```python
from build123d import *

# Parameters (mm, degrees)
SKETCH1_W           = 210
SKETCH1_H           = 210
SKETCH1_R           = 1.5
SKETCH1_R_2         = 10
SKETCH1_R_3         = 1.25
SKETCH1_W_2         = 30
SKETCH1_H_2         = 6.134133664
SKETCH1_H_3         = 6
SKETCH1_W_3         = 6.572229622
SKETCH1_H_4         = 24
SKETCH1_W_4         = 6
BOSS_EXTRUDE1_DEPTH = 6


with BuildPart() as part:
    # Sketch1 → Boss-Extrude1 (new body)
    with BuildSketch(Plane(origin=(0, 0, 0), x_dir=(1, 0, 0), z_dir=(0, 1, 0))):
        with Locations((-0.850910849, -4.383508225)):
            Rectangle(SKETCH1_W, SKETCH1_H)
        with Locations((-98.850910849, -90.383508225)):
            Circle(SKETCH1_R, mode=Mode.SUBTRACT)
        with Locations((-87.850910849, -90.383508225)):
            Circle(SKETCH1_R, mode=Mode.SUBTRACT)
        with Locations((-0.850910849, -60.383508225)):
            Circle(SKETCH1_R_2, mode=Mode.SUBTRACT)
        with Locations((-87.850910849, -30.383508225)):
            Circle(SKETCH1_R, mode=Mode.SUBTRACT)
        with Locations((-98.850910849, -30.383508225)):
            Circle(SKETCH1_R, mode=Mode.SUBTRACT)
        with Locations((97.149089151, -90.383508225)):
            Circle(SKETCH1_R, mode=Mode.SUBTRACT)
        with Locations((86.149089151, -90.383508225)):
            Circle(SKETCH1_R, mode=Mode.SUBTRACT)
        with Locations((86.149089151, -30.383508225)):
            Circle(SKETCH1_R, mode=Mode.SUBTRACT)
        with Locations((97.149089151, -30.383508225)):
            Circle(SKETCH1_R, mode=Mode.SUBTRACT)
        with Locations((-8.324910849, 80.616491775)):
            Circle(SKETCH1_R_3, mode=Mode.SUBTRACT)
        with Locations((6.623089151, 80.616491775)):
            Circle(SKETCH1_R_3, mode=Mode.SUBTRACT)
        with Locations((-35.350910849, 92.549424943)):
            Rectangle(SKETCH1_W_2, SKETCH1_H_2, mode=Mode.SUBTRACT)
        with Locations((-84.850910849, 92.616491775)):
            Rectangle(SKETCH1_W_2, SKETCH1_H_3, mode=Mode.SUBTRACT)
        with Locations((33.649089151, 92.549424943)):
            Rectangle(SKETCH1_W_2, SKETCH1_H_2, mode=Mode.SUBTRACT)
        with Locations((83.149089151, 92.616491775)):
            Rectangle(SKETCH1_W_2, SKETCH1_H_3, mode=Mode.SUBTRACT)
        with Locations((83.149089151, -101.383508225)):
            Rectangle(SKETCH1_W_2, SKETCH1_H_3, mode=Mode.SUBTRACT)
        with Locations((33.649089151, -101.316441393)):
            Rectangle(SKETCH1_W_2, SKETCH1_H_2, mode=Mode.SUBTRACT)
        with Locations((-35.350910849, -101.316441393)):
            Rectangle(SKETCH1_W_2, SKETCH1_H_2, mode=Mode.SUBTRACT)
        with Locations((-84.850910849, -101.383508225)):
            Rectangle(SKETCH1_W_2, SKETCH1_H_3, mode=Mode.SUBTRACT)
        with Locations((-96.564796038, 64.616491775)):
            Rectangle(SKETCH1_W_3, SKETCH1_H_4, mode=Mode.SUBTRACT)
        with Locations((-96.850910849, 16.616491775)):
            Rectangle(SKETCH1_W_4, SKETCH1_H_4, mode=Mode.SUBTRACT)
        with Locations((95.149089151, 16.616491775)):
            Rectangle(SKETCH1_W_4, SKETCH1_H_4, mode=Mode.SUBTRACT)
        with Locations((94.86297434, 64.616491775)):
            Rectangle(SKETCH1_W_3, SKETCH1_H_4, mode=Mode.SUBTRACT)
    extrude(amount=BOSS_EXTRUDE1_DEPTH)


solid = part.part
```
Could you check a few things on this model? Use its own coordinates, in mm. A direction names the side the tool comes from. Round coordinates to 2 decimals unless told otherwise and drop trailing zeros. Loops run counter-clockwise (first coordinate to the right, second up) from the corner with the lowest first, then second, coordinate; pieces in that order, holes last. Notation, with made-up numbers: M 57,77 L 107,77 A29 cw 107,110 Z; hole C 48,70.25 d7. An arc over 180 degrees is marked long. Write item = value, one per line.
1. I need wall thicknesses on probe 1 along Z at (x, y) = (-83, 5.2); probe 2 along X at (y, z) = (3.85, -62.5); probe 3 along Z at (x, y) = (-22.5, 5.8). Which ranges of each line are inside material? Lowest first, please.
Results below:
probe_1 = -100.62 to -95.62, -89.62 to 98.38, 104.38 to 109.38
probe_2 = -105.85 to -99.85, -93.28 to 91.58, 98.15 to 104.15
probe_3 = -100.62 to -95.62, -89.48 to 98.25, 104.38 to 109.38
2. I want a section at C-C, the plane y = 3.5. Count the separate pieces of the cut face and the enclosed holes in it, and give its area (3 significant figures).
Results below:
separate_pieces = 1
enclosed_holes = 23
area = 41,700 mm²
3. Thinking about a two-plate mould opening in Z: for faces 1 (the face through (-105.851, 3, 6)), 2 (the face through (-2, 3, 109.384)), 3 (the face through (-97, 3, -76.616)), which applies, +Z half, -Z half, draft (parallel to the pull), parting line (faces both ways), or undercut?
Results below:
face_1 = draft
face_2 = +Z half
face_3 = undercut
4. Which directions (+Z, -Z, +X, -X, +Y, -Y) give clear straight access to the entire face, cutting with the end or side of a thin tool? Please do faces 4 (the face through (-2, 6, 3)), 5 (the face through (-99.851, 3, -93)).
Results below:
face_4 = +Z, -Z, +X, -X, +Y
face_5 = +Y, -Y
5. I want a section at B-B, the plane z = -60.5. Write out the boundary of the cut face in (x, y), and give its area (3 significant figures).
Results below:
outline = M -105.85,0 L -99.85,0 L -99.85,6 L -105.85,6 Z; M -93.28,0 L 91.58,0 L 91.58,6 L -93.28,6 Z; M 98.15,0 L 104.15,0 L 104.15,6 L 98.15,6 Z
area = 1,180 mm²
6. I want a section at A-A, the plane x = 22. Write out the boundary of the cut face in (y, z).
Results below:
outline = M 0,-100.62 L 6,-100.62 L 6,-95.62 L 0,-95.62 Z; M 0,-89.48 L 6,-89.48 L 6,98.25 L 0,98.25 Z; M 0,104.38 L 6,104.38 L 6,109.38 L 0,109.38 Z
